Could you check a few things on this model? Use its own coordinates, in mm. A direction names the side the tool comes from. Round coordinates to 2 decimals unless told otherwise and drop trailing zeros. Loops run counter-clockwise (first coordinate to the right, second up) from the corner with the lowest first, then second, coordinate; pieces in that order, holes last.
from build123d import *

# Parameters (mm, degrees)
SKETCH1_W           = 64.008
SKETCH1_H           = 43.434
SKETCH1_W_2         = 58.928
SKETCH1_H_2         = 38.354
BOSS_EXTRUDE1_DEPTH = 12.7
SKETCH2_W           = 13.638305883
SKETCH2_H           = 43.434
BOSS_EXTRUDE2_DEPTH = 2.54
SKETCH3_R           = 1.327962253
SKETCH3_R_2         = 1.146659907
BOSS_EXTRUDE3_DEPTH = 2.54


with BuildPart() as part:
    # Sketch1 → Boss-Extrude1 (new body)
    with BuildSketch(Plane(origin=(0, 0, 0), x_dir=(1, 0, 0), z_dir=(0, 1, 0))):
        with Locations((-2.584823529, -0.216647059)):
            Rectangle(SKETCH1_W, SKETCH1_H)
        with Locations((-2.584823529, -0.216647059)):
            Rectangle(SKETCH1_W_2, SKETCH1_H_2, mode=Mode.SUBTRACT)
    extrude(amount=-BOSS_EXTRUDE1_DEPTH)

    # Sketch2 → Boss-Extrude2 (add)
    with BuildSketch(Plane.XZ.offset(12.7)):
        with Locations((-0.158376471, 0.216647059)):
            Rectangle(SKETCH2_W, SKETCH2_H)
    extrude(amount=BOSS_EXTRUDE2_DEPTH)

    # Sketch3 → Boss-Extrude3 (add)
    # profile 1 of 2: a face of its own
    with BuildSketch(Plane(origin=(0, 0, 0), x_dir=(1, 0, 0), z_dir=(0, 1, 0))):
        with BuildLine():
            ThreePointArc((-9.823823529, 21.500352941), (-14.039870548, 25.716399959), (-18.255917566, 21.500352941))
            Line((-18.255917566, 21.500352941), (-9.823823529, 21.500352941))
        make_face()
        with Locations(Location((-14.039870548, 23.532352941, 0), (0, 0, 270))):
            Circle(SKETCH3_R, mode=Mode.SUBTRACT)
    # profile 2 of 2: a face of its own
    with BuildSketch(Plane(origin=(0, 0, 0), x_dir=(1, 0, 0), z_dir=(0, 1, 0))):
        with BuildLine():
            ThreePointArc((-18.255917566, -21.933647059), (-14.039870548, -26.149694077), (-9.823823529, -21.933647059))
            Line((-9.823823529, -21.933647059), (-18.255917566, -21.933647059))
        make_face()
        with Locations(Location((-14.039870548, -23.965647059, 0), (0, 0, 270))):
            Circle(SKETCH3_R_2, mode=Mode.SUBTRACT)
    extrude(amount=-BOSS_EXTRUDE3_DEPTH)


solid = part.part
Item 1: We'd pull the mould along X, two halves only. Please class faces 1 (the flat face through (27.3, -12.7, -1.5)), 2 (the flat face through (-34.589, -6, 1)), 3 (the flat face through (26.879, -6, 0)): released by +X, released by -X, zero draft, split by the parting line, or undercut.
Results list:
face 1: zero draft
face 2: released by -X
face 3: undercut
Item 2: If we section it at B-B, the plane x = 17: Please give me the cut outline in (y, z).
Results list:
outline: (-12.7, -21.5) - (0, -21.5) - (0, -18.96) - (-12.7, -18.96) - close; (-12.7, 19.39) - (0, 19.39) - (0, 21.93) - (-12.7, 21.93) - close
Item 3: If I drill on line 1 along Z through (x, y) = (14.5, -9.25); line 2 along X through (y, z) = (-8, 5.5); line 3 along Y through (x, z) = (1, -11.5), over which ranges is the centre line in solid material (lowest first)?
Results list:
line 1: z = -21.5 to -18.96, 19.39 to 21.93
line 2: x = -34.59 to -32.05, 26.88 to 29.42
line 3: y = -15.24 to -12.7
Item 4: If we section it at D-D, the plane x = -5.5: Please give me the cut outline in (y, z), then the cut area to 3 significant figures.
Results list:
outline: (-15.24, -21.5) - (0, -21.5) - (0, -18.96) - (-12.7, -18.96) - (-12.7, 19.39) - (0, 19.39) - (0, 21.93) - (-15.24, 21.93) - close
area: 175 mm2
Item 5: For faces 4 (the flat face through (-32.049, -6, 0)), 5 (the flat face through (-14.1, -2.54, 22.6)), 6 (the flat face through (-13, -2.54, -22)), 7 (the flat face through (-3, -6, -18.96)), which set-ups out of +Z, -Z, +X, -X, +Y, -Y let a thin tool reach every point of the face, with its end or its side?
Results list:
face 4: +Y, -Y
face 5: +Z, +X, -X, -Y
face 6: -Z, +X, -X, -Y
face 7: +Y
Item 6: If we section it at A-A, the plane z = 6: Please give me the cut outline in (x, y).
Results list:
outline: (-34.59, -12.7) - (-32.05, -12.7) - (-32.05, 0) - (-34.59, 0) - close; (-6.98, -15.24) - (6.66, -15.24) - (6.66, -12.7) - (-6.98, -12.7) - close; (26.88, -12.7) - (29.42, -12.7) - (29.42, 0) - (26.88, 0) - close
Item 7: Will these pins go through, and if not, where does the flat tip stop? pin 1 (4.5 mm diameter, centred on x = -14.5, z = -23.5, fed in from -Y); pin 2 (1 mm diameter, centred on x = -9, y = -13, fed in from -Z); pin 3 (12 mm diameter, centred on x = 18.5, z = -13, fed in from +Y); pin 4 (4 mm diameter, centred on x = 2, z = -2, fed in from +Y).
Results list:
pin 1: stops at y = -12.7
pin 2: stops at z = -21.5
pin 3: stops at y = 0
pin 4: stops at y = -12.7
Item 8: If we section it at C-C, the plane y = -6: Please give me the cut outline in (x, z), then the cut area to 3 significant figures.
Results list:
outline: (-34.59, -21.5) - (29.42, -21.5) - (29.42, 21.93) - (-34.59, 21.93) - close; hole (-32.05, -18.96) - (26.88, -18.96) - (26.88, 19.39) - (-32.05, 19.39) - close
area: 520 mm2
